Geometry check sheet. Reference: the model listing, model coordinates, mm. A direction names the side the tool comes from. Coordinates: 2 decimals unless noted, no trailing zeros. Order: outer loops, then holes, each group sorted by start corner. A loop starts at its lowest first (then second) coordinate and runs counter-clockwise, first axis right, second up. Notation, with made-up numbers: (30, 34.5) - (52, 34.5) arc R19 cw to (52, 43.5) - close; hole circle Ø9 at (87.5, 54). An arc over 180 degrees is marked (long way). Return JSON: item names as keys, results as strings. Group by question number.
Item 1: Section check B-B on z = 25. Enter the section's corners in (x, y).
Item 2: Gauge pin test, flat ends, axial feed: pin 1 (15 mm diameter, centred on y = -24, z = 26, fed in from -X); pin 2 (9.5 mm diameter, centred on x = 39, y = -22.5, fed in from +Z); pin 3 (10 mm diameter, centred on x = 27, y = -24, fed in from +Z). Record the tip position at first contact, or that the pin passes through.
Item 3: Section check D-D on y = -4. Enter the section's corners in (x, z), then the cut area to 3 significant figures.
Item 4: Section check A-A on y = -23.5. Enter the section's corners in (x, z), then the cut area to 3 significant figures.
Item 5: Tool access check on faces 1 (the flat face through (24.2, -22.36, 22.09)), 2 (the flat face through (9, -22, 12.7)), 3 (the flat face through (40, -22, 12.7)). Record the directions out of +Z, -Z, +X, -X, +Y, -Y that give a thin tool (end or side, any length) a straight path to the whole face; none if there is none.
Item 6: Section check C-C on x = 13. Enter the section's corners in (y, z), then the cut area to 3 significant figures.
Item 7: Scan lines: probe 1 along X at (y, z) = (-17, 14); probe 2 along Y at (x, z) = (29.5, 13); probe 3 along Z at (x, y) = (48, -26). Record each from-to range of solid material in increasing order.
from build123d import *

# Parameters (mm, degrees)
F0_W     = 50.8
F0_H     = 31.75
F1_DEPTH = 31.75
F2_W     = 19.05
F2_H     = 19.05
F3_DEPTH = 19.05
F4_W     = 19.05
F4_H     = 19.05
F5_DEPTH = 21.59
F7_DEPTH = 25.4
F9_DEPTH = 25.4


with BuildPart() as f1:
    # F0 (on Front) → F1 (new body)
    with BuildSketch(Plane.XZ):
        with Locations((25.4, 15.875)):
            Rectangle(F0_W, F0_H)
    extrude(amount=F1_DEPTH)

    # F2 (on face) → F3 (cut)
    with BuildSketch(Plane(origin=(0, 0, 0), x_dir=(0, -1, 0), z_dir=(-1, 0, 0))):
        with Locations((22.225, 22.225)):
            Rectangle(F2_W, F2_H)
    extrude(amount=-F3_DEPTH, mode=Mode.SUBTRACT)

    # F4 (on face) → F5 (cut)
    with BuildSketch(Plane.YZ.offset(50.8)):
        with Locations((-22.225, 22.225)):
            Rectangle(F4_W, F4_H)
    extrude(amount=-F5_DEPTH, mode=Mode.SUBTRACT)

    # F6 (on face) → F7 (cut)
    with BuildSketch(Plane.YZ.offset(29.21)):
        Polygon((-31.75, 31.75), (-31.75, 12.7), (-12.7, 31.75), align=None)
    extrude(amount=-F7_DEPTH, mode=Mode.SUBTRACT)

    # F8 (on face) → F9 (cut)
    with BuildSketch(Plane(origin=(0, 0, 0), x_dir=(-1, 0, 0), z_dir=(0, 1, 0))):
        Polygon((-38.1, 31.75), (-50.8, 31.75), (-50.8, 12.7), align=None)
    extrude(amount=-F9_DEPTH, mode=Mode.SUBTRACT)


solid = f1.part
Computed:
{
 "1": {"outline": "(0, -12.7) - (19.05, -12.7) - (19.05, -19.45) - (29.21, -19.45) - (29.21, -12.7) - (42.6, -12.7) - (42.6, 0) - (0, 0) - close"},
 "2": {"pin 1": "stops at x = 19.05", "pin 2": "stops at z = 12.7", "pin 3": "stops at z = 25.45"},
 "3": {"outline": "(0, 0) - (50.8, 0) - (50.8, 12.7) - (38.1, 31.75) - (0, 31.75) - close", "area": "1,490 mm²"},
 "4": {"outline": "(0, 0) - (50.8, 0) - (50.8, 12.7) - (29.21, 12.7) - (29.21, 20.95) - (19.05, 20.95) - (19.05, 12.7) - (0, 12.7) - close", "area": "729 mm²"},
 "5": {"face 1": "+Z, +X, -X, -Y", "face 2": "+Z, -X, -Y", "face 3": "+Z, +X, -Y"},
 "6": {"outline": "(-31.75, 0) - (0, 0) - (0, 31.75) - (-12.7, 31.75) - (-12.7, 12.7) - (-31.75, 12.7) - close", "area": "645 mm²"},
 "7": {"probe 1": "x = 19.05 to 29.21", "probe 2": "y = -12.7 to 0", "probe 3": "z = 0 to 12.7"}
}
